Autodesk Inventor part; units mm, degrees
ref_plane "YZ Plane" through (0, 0, 0) normal (1, 0, 0) x (0, 1, 0)
ref_plane "XZ Plane" through (0, 0, 0) normal (0, 1, 0) x (-1, 0, 0)
ref_plane "XY Plane" through (0, 0, 0) normal (0, 0, 1) x (1, 0, 0)
sketch "Skizze1" plane through (0, 0, 0) normal (0, 0, 1) x (1, 0, 0)
  circle A0 centre (0, 0) radius 5
  circle A1 centre (0, 0) radius 8.5
  dimension "d0" = 10
  dimension "d1" = 17
extrude "Extrusion1" add sketch "Skizze1" along normal mid plane 30
sketch "Skizze2" plane through (0, 0, 0) normal (0, 0, 1) x (1, 0, 0)
  line L0 (0, 40.0774) -> (0, -42.4456) construction
  line L1 (-37.8898, 0) -> (75.0495, 0) construction
  circle A0 centre (0, 40) radius 30.5 construction
  circle A1 centre (0, 40) radius 30.5
  circle A2 centre (0, 0) radius 8.5
  line L2 (-4, 7.5) -> (-4, 9.7634)
  line L3 (4, 7.5) -> (4, 9.7634)
  circle A3 centre (0, 0) radius 8.5
  circle A4 centre (0, 40) radius 29
  line L4 (0, 40) -> (5.9896, 6.0311)
  line L5 (5.8214, 6.9852) -> (0, 40)
  line L6 (0, 40) -> (-5.9896, 6.0311)
  point P0 (-5.0358, 11.4406)
  point P1 (-5.9896, 6.0311)
  point P2 (5.9896, 6.0311)
  point P3 (5.0358, 11.4406)
  dimension "d4" = 61
  dimension "d5" = 40
  dimension "d6" = 8
  dimension "d7" = 1.5
  dimension "d8" = 10
  dimension "d9" = 10
extrude "Extrusion2" add sketch "Skizze2" along normal mid plane 30 contours A1 L6 A4 L4 | L2 A2 L6 A1 | A1 L3 A2 L2 | A1 L4 A2 L3 picked at (3.574, 10.751)
sketch "Skizze3" plane through (0, 0, 0) normal (1, 0, 0) x (0, 1, 0)
  line L0 (-8.5, -15) -> (-8.5, 15)
  line L1 (-8.5, -15) -> (6.0311, -15)
  arc A0 (-8.5, 0) -> (6.0311, -15) centre (5.1952, -1.2713) ccw
  line L2 (6.0311, -15) -> (-8.5, -15)
  line L3 (-8.5, -15) -> (-8.5, 0)
  point P0 (0, 0)
  point P1 (4.3593, -15)
  point P2 (-8.5, -2.5427)
extrude "Extrusion3" cut sketch "Skizze3" against normal mid plane 30 contours L0 A0 L1
mirror "Spiegeln1" about plane through (0, 0, 0) normal (0, 0, 1) of "Extrusion3"
properties part number "duct_round"
Input: part model. Units: mm. Frame: model coordinates. Coordinates: 2 decimals unless noted, no trailing zeros. Loops run counter-clockwise (first coordinate to the right, second up) from the corner with the lowest first, then second, coordinate; pieces in that order, holes last. Notation, with made-up numbers: M 12.5,62.5 L 20.5,62.5 A16 cw 20.5,88.5 Z; hole C 22.5,63.25 d1. An arc over 180 degrees is marked long. Answer in a Markdown table with one row per item.
1. First-contact query: pin 1 (1.5 mm diameter, centred on y = 0.5, z = -2.5, fed in from -X); pin 2 (1 mm diameter, centred on y = 9, z = -3, fed in from -X); pin 3 (3 mm diameter, centred on x = -3.5, z = -10.5, fed in from -Y); pin 4 (5 mm diameter, centred on y = 7.5, z = 7.5, fed in from -X). Flat tips, straight axial feed; report the tip coordinate or a pass-through.
Response:
| item | result |
|---|---|
| pin 1 | stops at x = -8.5 |
| pin 2 | stops at x = -5.55 |
| pin 3 | stops at y = -6.18 |
| pin 4 | stops at x = -6.87 |
2. Section B-B, the plane x = 0. Output: boundary loops of the cut face in (y, z), then the cut area to 3 significant figures.
Response:
| item | result |
|---|---|
| outline | M -8.5,-2.54 A13.75 ccw -5,-10.5 L -5,10.5 A13.75 ccw -8.5,2.54 Z; M 5,-15 L 11,-15 L 11,15 L 5,15 Z |
| area | 234 mm2 |
3. Section D-D, the plane z = -11. Output: boundary loops of the cut face in (x, y).
Response:
| item | result |
|---|---|
| outline | M -7.19,-4.53 L -2.12,-4.53 A5 cw long 2.12,-4.53 L 7.19,-4.53 A8.5 ccw 5.99,6.03 L 5.3,9.96 L 5.04,11.44 A29 cw -5.04,11.44 L -5.99,6.03 A8.5 ccw Z |
4. Section A-A, the plane z = 0.5. Output: boundary loops of the cut face in (x, y), then the cut area to 3 significant figures.
Response:
| item | result |
|---|---|
| outline | M -5.99,6.03 A8.5 ccw long 5.99,6.03 L 5.3,9.96 L 5.04,11.44 A29 cw -5.04,11.44 Z; hole C 0,0 d10 |
| area | 185 mm2 |
5. Section C-C, the plane y = -2.25. Output: boundary loops of the cut face in (x, z), then the cut area to 3 significant figures.
Response:
| item | result |
|---|---|
| outline | M -8.2,-12.84 L -4.47,-12.84 L -4.47,12.84 L -8.2,12.84 Z; M 4.47,-12.84 L 8.2,-12.84 L 8.2,12.84 L 4.47,12.84 Z |
| area | 192 mm2 |
6. Material intervals for line 1 (X direction, y = 0, z = 8.25); line 2 (Y direction, x = 1.5, z = 5); line 3 (Y direction, x = -2, z = 7), sorted ascending.
Response:
| item | result |
|---|---|
| line 1 | x = -8.5 to -5, 5 to 8.5 |
| line 2 | y = -8.04 to -4.77, 4.77 to 11.04 |
| line 3 | y = -7.31 to -4.58, 4.58 to 11.07 |
